The model under review builds one solid part; all positions refer to its coordinate system, in mm. Face numbers are marked on the shaded views. A direction names the side the tool comes from. Coordinates: 2 decimals unless noted, no trailing zeros. Order: outer loops, then holes, each group sorted by start corner. A loop starts at its lowest first (then second) coordinate and runs counter-clockwise, first axis right, second up. Notation, with made-up numbers: M 82.25,53 L 124.25,53 A7 cw 124.25,65 Z; hole C -1,53.25 d5. An arc over 180 degrees is marked long. Answer in a Markdown table with one row per item.
from build123d import *

# Parameters (mm, degrees)
F4_DEPTH      = 4
F4_DEPTH_BACK = 4


with BuildPart() as f1:
    # F0 (on Front) → F1 (revolve)
    with BuildSketch(Plane.XZ):
        Polygon((0, 6), (-5.1, 6), (-5.1, 0), (-3, 0), (-3, -24.385), (-2.385, -25), (0, -25), align=None)
    revolve(axis=Axis((0, 0, -9.5), (0, 0, -1)))

    # F3 (on offset) → F4 (cut, two sides)
    with BuildSketch(Plane.XY.offset(6)) as f4_sk:
        Polygon((2.5, -1.443376), (2.5, 1.443376), (0, 2.886751), (-2.5, 1.443376), (-2.5, -1.443376), (0, -2.886751), align=None)
    extrude(amount=-F4_DEPTH, mode=Mode.SUBTRACT)
    extrude(f4_sk.sketch, amount=-F4_DEPTH_BACK, mode=Mode.SUBTRACT)


solid = f1.part
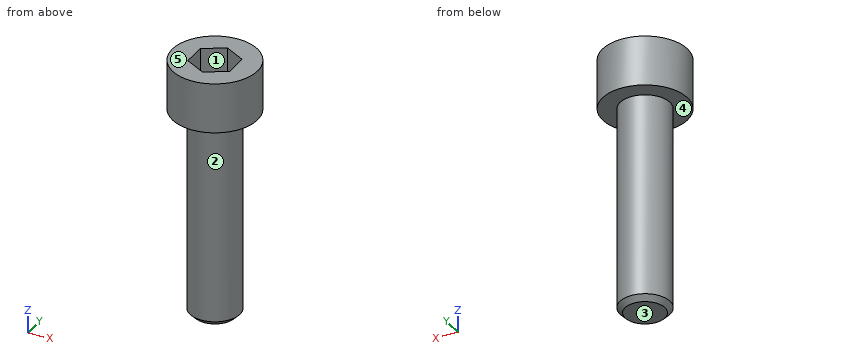
(1) Insertion check: P1, Ø6, axis at y = 0.5, z = -4.5, coming from the -X side. The pin has a flat end and moves straight along its axis. Give the tip position at first contact, or say it passes through.
Report:
| item | result |
|---|---|
| P1 | x = -3 |
(2) The part is to be moulded in two halves that separate along X. For the marked faces 1, 2 and 3, say which applies: +X half, -X half, draft (parallel to the pull), parting line (faces both ways), or undercut.
Report:
| item | result |
|---|---|
| face 1 | undercut |
| face 2 | parting line |
| face 3 | draft |
(3) Take a section at A-A (y = 0). Write out the cut boundary in (x, z) (3 decimals).
Report:
| item | result |
|---|---|
| outline | M -5.1,0 L -3,0 L -3,-24.385 L -2.385,-25 L 2.385,-25 L 3,-24.385 L 3,0 L 5.1,0 L 5.1,6 L 2.5,6 L 2.5,2 L -2.5,2 L -2.5,6 L -5.1,6 Z |
(4) Take a section at B-B (z = -19). Write out the cut boundary in (x, y).
Report:
| item | result |
|---|---|
| outline | C 0,0 d6 |
(5) Take a section at C-C (x = -4). Write out the cut boundary in (y, z), then the cut area to 3 significant figures.
Report:
| item | result |
|---|---|
| outline | M -3.16,0 L 3.16,0 L 3.16,6 L -3.16,6 Z |
| area | 38.0 mm^2 |
(6) To check wall thickness, follow line 1 (Z direction, x = 2, y = -2.75); line 2 (Z direction, x = 0.75, y = -0.75); line 3 (Y direction, x = 0, z = -16). State the ranges of each line that lie inside material, in increasing order. Write a range as [from, to].
Report:
| item | result |
|---|---|
| line 1 | [0, 6] |
| line 2 | [-25, 2] |
| line 3 | [-3, 3] |
(7) Machinability: for the marked faces 4 and 5, which of the approach directions +Z, -Z, +X, -X, +Y, -Y give a long, thin tool a straight path to every point of the face, cutting with its end or side? Answer none if there is none.
Report:
| item | result |
|---|---|
| face 4 | -Z |
| face 5 | +Z, +X, -X, +Y, -Y |
